from build123d import *

# Parameters (mm, degrees)
EXTRUDE_6_DEPTH      = 39
CUT_EXTRUDE_START    = 3
CUT_EXTRUDE_2_DEPTH  = 33
EXTRUDE_START        = 9.5
SKETCH_7_W           = 35
SKETCH_7_H           = 13
EXTRUDE_7_DEPTH      = 20
EXTRUDE_START_2      = 4.5
SKETCH_11_W          = 17
SKETCH_11_H          = 2.5
EXTRUDE_15_DEPTH     = 30
CUT_EXTRUDE_START_2  = 180
CUT_EXTRUDE_3_DEPTH  = 10
SKETCH_13_R          = 1.5
CUT_EXTRUDE_4_DEPTH  = 30
SKETCH_14_W          = 15
SKETCH_14_H          = 2
CUT_EXTRUDE_5_DEPTH  = 30
CUT_EXTRUDE_START_3  = 17
CUT_EXTRUDE_7_DEPTH  = 85
CUT_EXTRUDE_START_4  = 13
CUT_EXTRUDE_9_DEPTH  = 5
SKETCH_20_W          = 16.6
SKETCH_20_H          = 24.7
CUT_EXTRUDE_10_DEPTH = 5
SKETCH_21_R          = 6
CUT_EXTRUDE_11_DEPTH = 5


with BuildPart() as part:
    # Эскиз1 → Бобышка-Вытянуть6 (new body)
    with BuildSketch(Plane.XY):
        with BuildLine():
            Line((4.299618531, 175.402841826), (4.299618531, 188.402841826))
            Line((4.299618531, 188.402841826), (75.299618531, 188.402841826))
            Line((75.299618531, 188.402841826), (96.299618531, 168.402841826))
            Line((96.299618531, 168.402841826), (96.299619, 0))
            Line((96.299619, 0), (96.299619, -28))
            Line((96.299619, -28), (0, -28))
            Line((0, -28), (0, 0))
            ThreePointArc((0, 0), (37.229295141, 21.561020186), (55.173142182, 60.662380285))
            ThreePointArc((55.173142182, 60.662380285), (56.797307883, 87.162380285), (55.173142182, 113.662380285))
            ThreePointArc((55.173142182, 113.662380285), (38.726552267, 151.940422917), (4.299618531, 175.402841826))
        make_face()
    extrude(amount=EXTRUDE_6_DEPTH)

    # Эскиз5 → Вырез-Вытянуть2 (cut)
    with BuildSketch(Plane.XY.offset(CUT_EXTRUDE_START)):
        Polygon((34.099618531, 175.402841826), (4.299618531, 175.402841826), (4.299618531, 169.021888999), (-18.700381469, 169.021888999), (-18.700381469, -25), (14, -25), (14, 6.5), (30.299619, 6.5), (30.299619, -25), (91.299619, -25), (91.299619, 169.021888999), (74.099618531, 185.402841826), (34.099618531, 185.402841826), align=None)
    extrude(amount=CUT_EXTRUDE_2_DEPTH, mode=Mode.SUBTRACT)

    # Эскиз7 → Бобышка-Вытянуть7 (add)
    with BuildSketch(Plane.XY.offset(EXTRUDE_START)):
        with Locations((-13.200381469, 181.902841826)):
            Rectangle(SKETCH_7_W, SKETCH_7_H)
    extrude(amount=EXTRUDE_7_DEPTH)

    # Эскиз11 → Бобышка-Вытянуть15 (add)
    with BuildSketch(Plane.XY.offset(EXTRUDE_START_2)):
        with Locations((-2.200381469, 174.152841826)):
            Rectangle(SKETCH_11_W, SKETCH_11_H)
    extrude(amount=EXTRUDE_15_DEPTH)

    # Эскиз12 → Вырез-Вытянуть3 (cut)
    with BuildSketch(Plane(origin=(0, 0, 0), x_dir=(1, 0, 0), z_dir=(0, 1, 0)).offset(CUT_EXTRUDE_START_2)):
        with BuildLine():
            Line((-7.700381469, -34.154700538), (-7.200381469, -33.866025404))
            ThreePointArc((-7.200381469, -33.866025404), (-7.700381469, -32), (-8.200381469, -33.866025404))
            Line((-8.200381469, -33.866025404), (-7.700381469, -34.154700538))
        make_face()
        with BuildLine():
            Line((-7.700381469, -7.154700538), (-7.200381469, -6.866025404))
            ThreePointArc((-7.200381469, -6.866025404), (-7.700381469, -5), (-8.200381469, -6.866025404))
            Line((-8.200381469, -6.866025404), (-7.700381469, -7.154700538))
        make_face()
    extrude(amount=-CUT_EXTRUDE_3_DEPTH, mode=Mode.SUBTRACT)

    # Эскиз13 → Вырез-Вытянуть4 (cut)
    with BuildSketch(Plane.XY):
        with Locations((-2.700381469, 183.402841826)):
            Circle(SKETCH_13_R)
    extrude(amount=CUT_EXTRUDE_4_DEPTH, mode=Mode.SUBTRACT)

    # Эскиз14 → Вырез-Вытянуть5 (cut)
    with BuildSketch(Plane.XY):
        with Locations((-23.200381469, 187.402841826)):
            Rectangle(SKETCH_14_W, SKETCH_14_H)
    extrude(amount=CUT_EXTRUDE_5_DEPTH, mode=Mode.SUBTRACT)

    # Эскиз17 → Вырез-Вытянуть7 (cut)
    with BuildSketch(Plane(origin=(0, 0, 0), x_dir=(0, 0, -1), z_dir=(1, 0, 0)).offset(CUT_EXTRUDE_START_3)):
        with BuildLine():
            Line((-24.118802154, -2.5), (-22.964101615, -0.5))
            ThreePointArc((-22.964101615, -0.5), (-15.5, -2.5), (-22.964101615, -4.5))
            Line((-22.964101615, -4.5), (-24.118802154, -2.5))
        make_face()
    extrude(amount=CUT_EXTRUDE_7_DEPTH, mode=Mode.SUBTRACT)

    # Эскиз18 → Вырез-Вытянуть9 (cut)
    with BuildSketch(Plane(origin=(0, 0, 0), x_dir=(0, 0, -1), z_dir=(1, 0, 0)).offset(CUT_EXTRUDE_START_4)):
        with BuildLine():
            Line((-21.809401077, -2.5), (-21.232050808, -1.5))
            ThreePointArc((-21.232050808, -1.5), (-17.5, -2.5), (-21.232050808, -3.5))
            Line((-21.232050808, -3.5), (-21.809401077, -2.5))
        make_face()
    extrude(amount=CUT_EXTRUDE_9_DEPTH, mode=Mode.SUBTRACT)

    # Эскиз20 → Вырез-Вытянуть10 (cut)
    with BuildSketch(Plane(origin=(0, 188.402841826, 0), x_dir=(1, 0, 0), z_dir=(0, 1, 0))):
        with Locations((40.95, -19.5)):
            Rectangle(SKETCH_20_W, SKETCH_20_H)
        with BuildLine():
            Line((30, -32.143375673), (30.625, -31.782531755))
            ThreePointArc((30.625, -31.782531755), (30, -29.45), (29.375, -31.782531755))
            Line((29.375, -31.782531755), (30, -32.143375673))
        make_face()
        with BuildLine():
            Line((30, -9.743375673), (30.625, -9.382531755))
            ThreePointArc((30.625, -9.382531755), (30, -7.05), (29.375, -9.382531755))
            Line((29.375, -9.382531755), (30, -9.743375673))
        make_face()
        with BuildLine():
            Line((51.9, -9.743375673), (52.525, -9.382531755))
            ThreePointArc((52.525, -9.382531755), (51.9, -7.05), (51.275, -9.382531755))
            Line((51.275, -9.382531755), (51.9, -9.743375673))
        make_face()
        with BuildLine():
            Line((51.9, -32.143375673), (52.525, -31.782531755))
            ThreePointArc((52.525, -31.782531755), (51.9, -29.45), (51.275, -31.782531755))
            Line((51.275, -31.782531755), (51.9, -32.143375673))
        make_face()
    extrude(amount=-CUT_EXTRUDE_10_DEPTH, mode=Mode.SUBTRACT)

    # Эскиз21 → Вырез-Вытянуть11 (cut)
    with BuildSketch(Plane(origin=(129.903734815, 136.398921556, 0), x_dir=(0, 0, -1), z_dir=(0.689655172, 0.724137931, 0))):
        with Locations((-19.5, 60.905684392)):
            Circle(SKETCH_21_R)
    extrude(amount=-CUT_EXTRUDE_11_DEPTH, mode=Mode.SUBTRACT)


solid = part.part
The listing builds one solid part. Answer for the finished solid, in the listing's coordinates (mm). A direction names the side the tool comes from. Coordinates: 2 decimals unless noted, no trailing zeros. Write each loop counter-clockwise with the first axis right and the second up, starting at its lowest first coordinate (ties: lowest second). Pieces come first, ordered by that corner, then holes. Notation, with made-up numbers: M 0,80.25 L 51,80.25 A9 cw 51,94.25 Z; hole C 16.5,25 d10. An arc over 180 degrees is marked long. Write each question's results on one line, items separated by ' | '.
Item 1: Which of the six approach directions +Z, -Z, +X, -X, +Y, -Y give full straight-line access (tool end or side, diameter ignored) to faces 1 (the face through (91.3, 71, 19)), 2 (the face through (32.51, 16.84, 36.74)), 3 (the face through (-3, 175.403, 7))?
Answer below:
face 1: none | face 2: +Z, -Z, -X | face 3: -Z, -X, +Y
Item 2: The part is cut by section A-A on x = 42. Determine the outline of the cut face in (y, z), and give its area (3 significant figures).
Answer below:
outline: M -28,0 L 27.4,0 L 27.4,3 L -25,3 L -25,36 L 27.4,36 L 27.4,39 L -28,39 Z; M 147.66,0 L 188.4,0 L 188.4,7.15 L 185.4,7.15 L 185.4,3 L 147.66,3 Z; M 147.66,36 L 185.4,36 L 185.4,31.85 L 188.4,31.85 L 188.4,39 L 147.66,39 Z | area: 701 mm2
Item 3: The part is cut by section B-B on y = 85. Determine the outline of the cut face in (x, z), and give its area (3 significant figures).
Answer below:
outline: M 56.79,0 L 96.3,0 L 96.3,39 L 56.79,39 L 56.79,36 L 91.3,36 L 91.3,3 L 56.79,3 Z | area: 402 mm2
Item 4: The part is cut by section C-C on y = 18. Determine the outline of the cut face in (x, z), and give its area (3 significant figures).
Answer below:
outline: M 33.75,0 L 96.3,0 L 96.3,39 L 33.75,39 L 33.75,36 L 91.3,36 L 91.3,3 L 33.75,3 Z | area: 540 mm2
Item 5: For a pull along Y with two mould halves and no side action, classify faces 4 (the face through (39.101, 151.483, 1.479)), 5 (the face through (-13, 182, 29.5)), 6 (the face through (-23, 186.403, 19)) as released by +Y, released by -Y, zero draft, split by the parting line, or undercut.
Answer below:
face 4: undercut | face 5: zero draft | face 6: released by +Y
Item 6: Consider probe 1 along Z at (x, y) = (30, 186); probe 2 along Y at (x, z) = (25.25, 19.5); probe 3 along Y at (x, z) = (64, 6). Determine where each line is inside the solid, lowest interval first. Write a range as [from, to].
Answer below:
probe 1: [0, 7.05], [9.74, 29.45], [32.14, 39] | probe 2: [-28, -6.5], [1.5, 6.5], [175.4, 188.4] | probe 3: [-28, -25], [185.4, 188.4]
Item 7: Given P1, Ø7.5, axis at x = -23, z = 19.5, coming from the +Y side; P2, Ø15, axis at y = -9, z = 22, coming from the -X side; P3, Ø1, axis at y = 103, z = 10.5, coming from the -X side, each flat-ended and moving along its own axis, determine where each tip first touches the part or whether it passes through.
Answer below:
P1: y = 186.4 | P2: x = 14 | P3: x = 91.3
